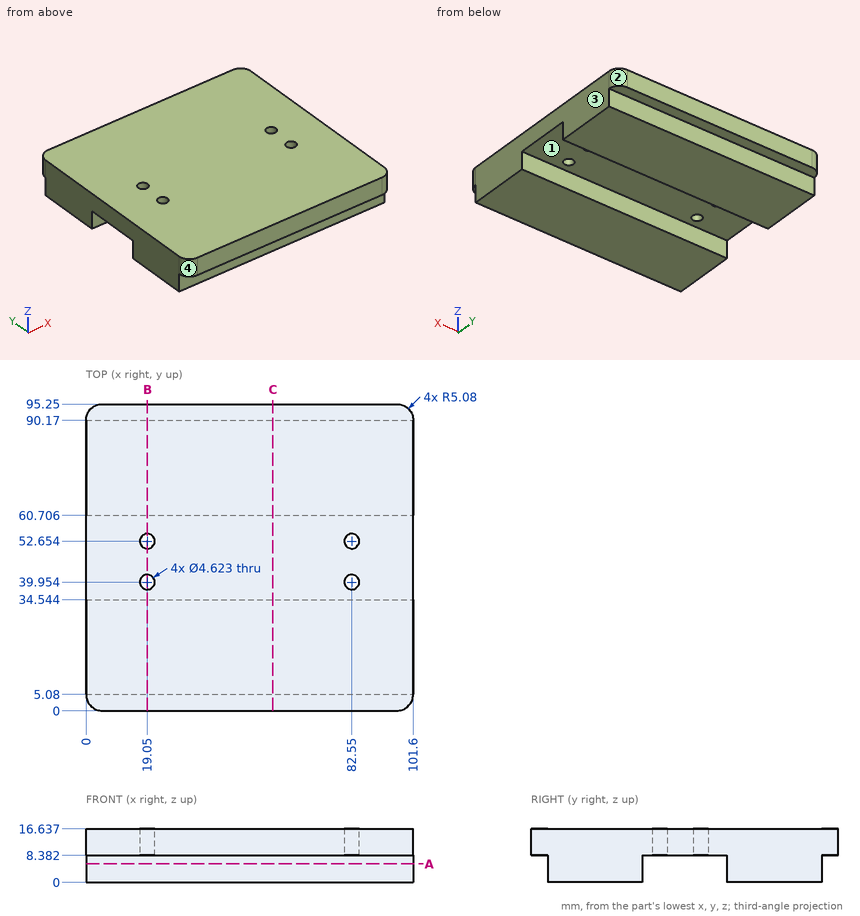
Design review of the part shown in the three views and the two pictorial views. Dimensions are in mm from the part's minimum x, y and z. Round coordinates to 2 decimals unless told otherwise and drop trailing zeros. Loops run counter-clockwise (first coordinate to the right, second up) from the corner with the lowest first, then second, coordinate; pieces in that order, holes last.
1) Consider section B-B on x = 19.05. State the section outline as (y, z) points.
Values follow:
outline: (0, 8.38) - (5.08, 8.38) - (5.08, 0) - (34.54, 0) - (34.54, 8.38) - (37.64, 8.38) - (37.64, 16.64) - (0, 16.64) - close; (42.27, 8.38) - (50.34, 8.38) - (50.34, 16.64) - (42.27, 16.64) - close; (54.97, 8.38) - (60.71, 8.38) - (60.71, 0) - (90.17, 0) - (90.17, 8.38) - (95.25, 8.38) - (95.25, 16.64) - (54.97, 16.64) - close
2) The part is to be moulded in two halves that separate along Y. For the marked faces 1, 2, 3 and 4, say which applies: pulls with the +Y half, pulls with the -Y half, needs draft (parallel to the pull), parting line crosses it, or undercut.
Values follow:
face 1: undercut
face 2: pulls with the +Y half
face 3: needs draft
face 4: pulls with the -Y half
3) Clearance check with flat-ended pins moving along their axes: P1, Ø21, axis at x = 72.5, y = 47, coming from the -Z side; P2, Ø1.5, axis at x = 85.5, z = 7.5, coming from the -Y side; P3, Ø3, axis at x = 19.05, y = 52.65, coming from the -Z side; P4, Ø8, axis at x = 38.5, z = 3, coming from the +Y side. State where each tip first meets the part, or that it passes through.
Values follow:
P1: stops at z = 8.38
P2: stops at y = 5.08
P3: passes through
P4: stops at y = 90.17
4) Consider section C-C on x = 58. State the section outline as (y, z) points.
Values follow:
outline: (0, 8.38) - (5.08, 8.38) - (5.08, 0) - (34.54, 0) - (34.54, 8.38) - (60.71, 8.38) - (60.71, 0) - (90.17, 0) - (90.17, 8.38) - (95.25, 8.38) - (95.25, 16.64) - (0, 16.64) - close
5) Consider section A-A on z = 5.75. State the section outline as (x, y) points, then the cut area to 3 significant figures.
Values follow:
outline: (0, 5.08) - (101.6, 5.08) - (101.6, 34.54) - (0, 34.54) - close; (0, 60.71) - (101.6, 60.71) - (101.6, 90.17) - (0, 90.17) - close
area: 5,990 mm2
6) Wall thickness on line 1 along X through (y, z) = (40, 10); line 2 along Y through (x, z) = (82.55, 11.5); line 3 along Y through (x, z) = (6, 6.25): over which ranges is each line inside the solid? List them lowest first.
Values follow:
line 1: x = 0 to 16.74, 21.36 to 80.24, 84.86 to 101.6
line 2: y = 0 to 37.64, 42.27 to 50.34, 54.97 to 95.25
line 3: y = 5.08 to 34.54, 60.71 to 90.17
